Here's the drawing with two shaded views (mm, measured from the low corner). I have some questions. A direction names the side the tool comes from. Round coordinates to 2 decimals unless told otherwise and drop trailing zeros. Order: outer loops, then holes, each group sorted by start corner. A loop starts at its lowest first (then second) coordinate and runs counter-clockwise, first axis right, second up. Notation, with made-up numbers: (17, 59) -> (73, 59) arc R12 ccw to (73, 78) -> close; hole circle Ø6 at (-22.5, 16.25). An arc over 180 degrees is marked (long way). One line per question, with ' | ' between items.
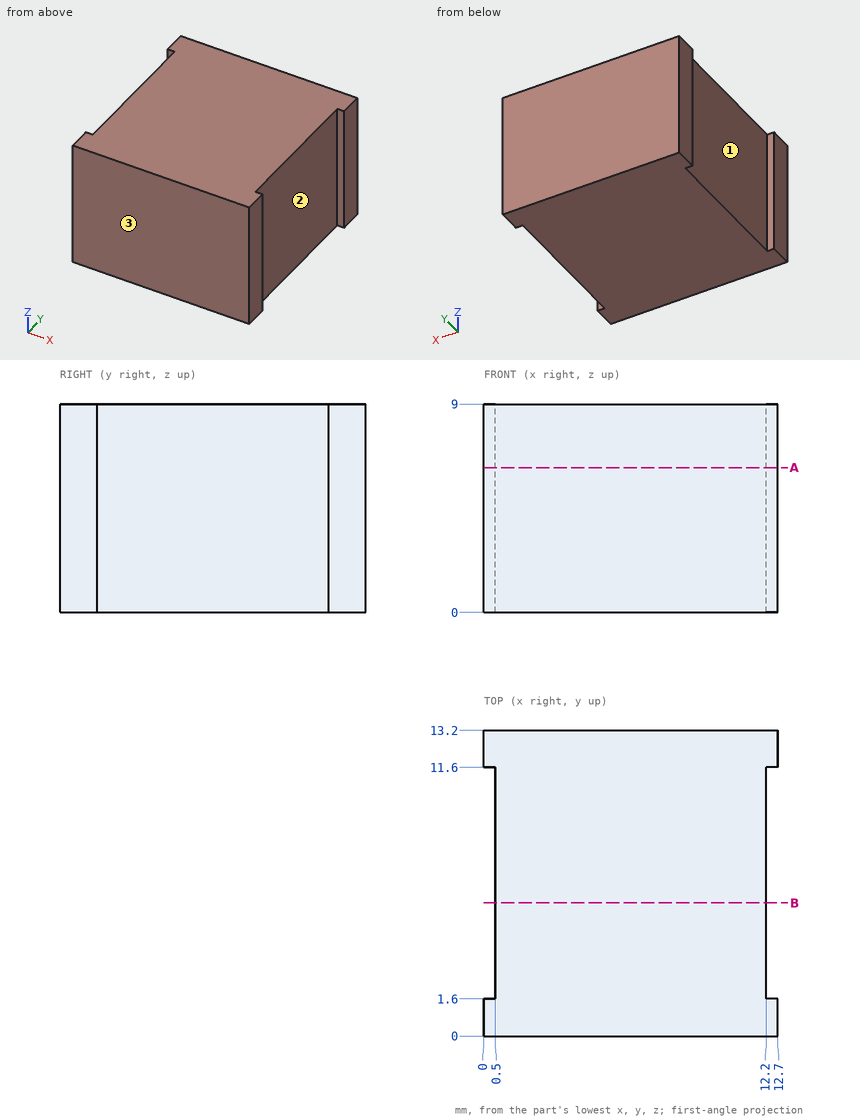
1. I need wall thicknesses on probe 1 along X at (y, z) = (9, 3). Which ranges of the line are inside material? Lowest first, please.
From the geometry:
probe 1: x = 0.5 to 12.2
2. I'm going to push flat-ended pins straight in: pin 1 (2.5 mm diameter, centred on y = 7.5, z = 5.5, fed in from +X); pin 2 (2.5 mm diameter, centred on y = 6.5, z = 3.5, fed in from -X). Where does each tip first touch, or does it pass through?
From the geometry:
pin 1: stops at x = 12.2 | pin 2: stops at x = 0.5
3. I want a section at B-B on y = 5.75. List the corners of the cut face in (x, z) for me, and give its area (3 significant figures).
From the geometry:
outline: (0.5, 0) -> (12.2, 0) -> (12.2, 9) -> (0.5, 9) -> close | area: 105 mm²
4. On a 3-axis mill with a long thin cutter (end or side, diameter ignored), from which of +Z, -Z, +X, -X, +Y, -Y can I reach the whole of each face in a straight line? I mean the marked faces 1, 2 and 3. Say none if no direction works.
From the geometry:
face 1: +Z, -Z, -X | face 2: +Z, -Z, +X | face 3: +Z, -Z, +X, -X, -Y
5. I want a section at A-A on z = 6.25. List the corners of the cut face in (x, y) for me, and give its area (3 significant figures).
From the geometry:
outline: (0, 0) -> (12.7, 0) -> (12.7, 1.6) -> (12.2, 1.6) -> (12.2, 11.6) -> (12.7, 11.6) -> (12.7, 13.2) -> (0, 13.2) -> (0, 11.6) -> (0.5, 11.6) -> (0.5, 1.6) -> (0, 1.6) -> close | area: 158 mm²
